from build123d import *

# Parameters (mm, degrees)
F0_R     = 1.5
F1_DEPTH = 5


with BuildPart() as f1:
    # F0 (on Right) → F1 (new body)
    with BuildSketch(Plane.YZ):
        with BuildLine():
            Line((80.000096, 25.85796), (97.071068, 42.928932))
            ThreePointArc((97.071068, 42.928932), (97.071068, 57.071068), (82.928932, 57.071068))
            Line((82.928932, 57.071068), (65.857864, 40))
            ThreePointArc((65.857864, 40), (-1.379349, 26.831799), (-65.857864, 50))
            Line((-65.857864, 50), (-82.928932, 67.071068))
            ThreePointArc((-82.928932, 67.071068), (-97.071068, 67.071068), (-97.071068, 52.928932))
            Line((-97.071068, 52.928932), (-80.000096, 35.85796))
            ThreePointArc((-80.000096, 35.85796), (-65.147242, 0), (-80.000096, -35.85796))
            Line((-80.000096, -35.85796), (-97.071068, -52.928932))
            ThreePointArc((-97.071068, -52.928932), (-97.071068, -67.071068), (-82.928932, -67.071068))
            Line((-82.928932, -67.071068), (-65.857864, -50))
            ThreePointArc((-65.857864, -50), (-1.379349, -26.831799), (65.857864, -40))
            Line((65.857864, -40), (82.928932, -57.071068))
            ThreePointArc((82.928932, -57.071068), (97.071068, -57.071068), (97.071068, -42.928932))
            Line((97.071068, -42.928932), (80.000096, -25.85796))
            ThreePointArc((80.000096, -25.85796), (69.289378, 0), (80.000096, 25.85796))
        make_face()
        with Locations((-55.858192, -25.85796)):
            Circle(F0_R, mode=Mode.SUBTRACT)
        with BuildLine():
            ThreePointArc((64.35796, -25.85796), (65.85796, -24.35796), (67.35796, -25.85796))
            ThreePointArc((67.35796, -25.85796), (65.85796, -27.35796), (64.35796, -25.85796))
        make_face(mode=Mode.SUBTRACT)
        with Locations((-55.858192, 25.85796)):
            Circle(F0_R, mode=Mode.SUBTRACT)
        with Locations((65.85796, 25.85796)):
            Circle(F0_R, mode=Mode.SUBTRACT)
    extrude(amount=F1_DEPTH)


solid = f1.part
Could you check a few things on this model? Use its own coordinates, in mm. A direction names the side the tool comes from. Give positions to 0.01 mm unless a question says otherwise; leave off trailing zeros. Write each loop counter-clockwise with the first axis right and the second up, starting at its lowest first coordinate (ties: lowest second). Pieces come first, ordered by that corner, then holes. Notation, with made-up numbers: (-35.75, 59.5) - (20.25, 59.5) arc R11 ccw to (20.25, 63.5) - close; hole circle Ø6 at (-37.75, -8.75). An arc over 180 degrees is marked (long way). Use CSV: the item, a comma, the result in double quotes. Start each with the question number.
Item 1: I want a section at B-B, the plane x = 2.25. Please give me the cut outline in (y, z).
Item 2: I want a section at D-D, the plane y = 9.5. Please give me the cut outline in (x, z).
Item 3: I want a section at A-A, the plane y = -90. Please give me the cut outline in (x, z), then the cut area to 3 significant figures.
Item 4: For faces 5 (the face through (2.465, -74.513, -58.655)), 6 (the face through (2.465, -74.274, 58.416)), 7 (the face through (2.465, -88.655, 44.513)), which set-ups out of +Z, -Z, +X, -X, +Y, -Y let a thin tool reach every point of the face, with its end or its side?
Item 5: I'm going to push flat-ended pins straight in: pin 1 (1.8 mm diameter, centred on y = -55.86, z = 25.86, fed in from +X); pin 2 (3 mm diameter, centred on x = 1.5, z = 19.5, fed in from -Y); pin 3 (3 mm diameter, centred on x = 3, y = -40.5, fed in from +Z); pin 4 (3.5 mm diameter, centred on y = 65.86, z = -25.86, fed in from +X). Where does each tip first touch, or does it pass through?
Item 6: If I drill on line 1 along Y through (x, z) = (1.85, 26); line 2 along Y through (x, z) = (1.95, 25.5) (3 decimals); line 3 along Z through (x, y) = (2.4, 82), over which ranges is the centre line in solid material (lowest first)?
Item 7: I want a section at C-C, the plane z = -19. Please give me the cut outline in (x, y), then the cut area to 3 significant figures.
Item 8: If we mould it in two halves opening along Y, with no side actions, what happens to faces 1 (the face through (2.465, 88.416, 34.274)), 2 (the face through (2.46, -2.35, -26.91)), 3 (the face through (2.465, -88.416, -44.274)), 4 (the face through (2.46, -0.41, 26.76))? For each: pulls with the +Y half, pulls with the -Y half, needs draft (parallel to the pull), parting line crosses it, or undercut.
Findings:
1,outline,"(-97.07, -52.93) arc R10 ccw to (-82.93, -67.07) - (-65.86, -50) arc R128.82 cw to (65.86, -40) - (82.93, -57.07) arc R10 ccw to (97.07, -42.93) - (80, -25.86) arc R36.57 cw to (80, 25.86) - (97.07, 42.93) arc R10 ccw to (82.93, 57.07) - (65.86, 40) arc R128.82 cw to (-65.86, 50) - (-82.93, 67.07) arc R10 ccw to (-97.07, 52.93) - (-80, 35.86) arc R50.71 cw to (-80, -35.86) - close; hole circle Ø3 at (-55.86, -25.86); hole circle Ø3 at (-55.86, 25.86); hole circle Ø3 at (65.86, -25.86); hole circle Ø3 at (65.86, 25.86)"
2,outline,"(0, -26.47) - (5, -26.47) - (5, 26.47) - (0, 26.47) - close"
3,outline,"(0, -70) - (5, -70) - (5, -45.86) - (0, -45.86) - close; (0, 45.86) - (5, 45.86) - (5, 70) - (0, 70) - close"
3,area,"241 mm2"
4,face 5,"-Z, +X, -X"
4,face 6,"+Z, +X, -X"
4,face 7,"+X, -X, -Y"
5,pin 1,"passes through"
5,pin 2,"stops at y = -69.7"
5,pin 3,"stops at z = 36.72"
5,pin 4,"stops at x = 5"
6,line 1,"y = -72.32 to -57.35, -54.36 to 64.36, 67.35 to 80.14"
6,line 2,"y = -72.025 to -57.315, -54.402 to 64.401, 67.315 to 79.647"
6,line 3,"z = -56.14 to -27.86, 27.86 to 56.14"
7,outline,"(0, -68.84) - (5, -68.84) - (5, 74.61) - (0, 74.61) - close"
7,area,"717 mm2"
8,face 1,"pulls with the +Y half"
8,face 2,"undercut"
8,face 3,"pulls with the -Y half"
8,face 4,"undercut"
